```python
from build123d import *

# Parameters (mm, degrees)
SKETCH1_R           = 10
BOSS_EXTRUDE1_DEPTH = 35
SKETCH2_R           = 2.9
CUT_EXTRUDE1_DEPTH  = 12
CUT_EXTRUDE1_DRAFT  = 1
SKETCH4_R           = 2.38125
CUT_EXTRUDE2_DEPTH  = 35
SKETCH5_R           = 2.8
CUT_EXTRUDE3_DEPTH  = 38.749172176


with BuildPart() as part:
    # Sketch1 → Boss-Extrude1 (new body)
    with BuildSketch(Plane.XY):
        Circle(SKETCH1_R)
    extrude(amount=BOSS_EXTRUDE1_DEPTH)


with BuildPart() as cut_extrude1_tool:
    # Sketch2 → Cut-Extrude1 (with draft: the straight prism first)
    with BuildSketch(Plane.XY.offset(12)):
        Circle(SKETCH2_R)
    extrude(amount=-CUT_EXTRUDE1_DEPTH)
    # Cut-Extrude1: the draft: its side faces are tilted about the plane it starts from
    cut_extrude1_sides = [cut_extrude1_tool.faces().sort_by_distance(p)[0] for p in [
        (-2.9, 0, 6),
    ]]
    draft(cut_extrude1_sides, Plane.XY.offset(12), CUT_EXTRUDE1_DRAFT)


with BuildPart() as part_1:
    add(part.part)

    # Cut-Extrude1: cut by cut_extrude1_tool
    add(cut_extrude1_tool.part, mode=Mode.SUBTRACT)

    # Sketch4 → Cut-Extrude2 (cut)
    with BuildSketch(Plane.XY.offset(35)):
        Circle(SKETCH4_R)
    extrude(amount=-CUT_EXTRUDE2_DEPTH, mode=Mode.SUBTRACT)

    # Sketch5 → Cut-Extrude3 (cut, through all)
    with BuildSketch(Plane(origin=(0, 0, 0), x_dir=(1, 0, 0), z_dir=(0, 1, 0))):
        with Locations(Location((0, -7, 0), (0, 0, 90))):
            Circle(SKETCH5_R)
    extrude(amount=CUT_EXTRUDE3_DEPTH, mode=Mode.SUBTRACT)


solid = part_1.part
```
Build history of the part. All positions in model axes, mm. A direction names the side the tool comes from. Give positions to 0.01 mm unless a question says otherwise; leave off trailing zeros. Loops run counter-clockwise (first coordinate to the right, second up) from the corner with the lowest first, then second, coordinate; pieces in that order, holes last. Notation, with made-up numbers: (-37.5, 9) -> (0.5, 9) arc R6 cw to (0.5, 16) -> close; hole circle Ø4 at (17.5, 85.25). An arc over 180 degrees is marked (long way). One line per question, with ' | ' between items. Start each with the question number.
1) Pin check, flat tip, straight feed: pin 1 (3 mm diameter, centred on x = 3, z = 12.5, fed in from +Y). Stop position of the tip, or through.
2) Cut at A-A (z = 29). Give the cut face in (x, y).
3) Two-plate mould, pull along Y, no slides. Class faces 3 (the flat face through (-2.4, 2.4, 0)), 4 (the cylindrical face through (-2.17, -9.76, 17.26)), 5 (the conical face through (-0.651, -2.932, 6.084)): released by +Y, released by -Y, zero draft, split by the parting line, or undercut.
4) Cut at D-D (y = -4.5). Give the cut face in (x, z), plus the area to 3 significant figures.
5) Cut at C-C (x = 0). Count the separate pieces of the cut face and the enclosed holes in it, plus the area to 3 significant figures.
6) 3-axis set-ups, long thin cutter, end or side, ignore diameter. For faces 1 (the cylindrical face through (-0.1, 6.5, 9.8)), 2 (the flat face through (2, -2, 35)): which of +Z, -Z, +X, -X, +Y, -Y reach the whole face in a straight line?
7) Cut at B-B (y = 3.5). Give the cut face in (x, z), plus the area to 3 significant figures.
8) Probe L1, parallel to Y at x = 1.5, z = 33.5; L2, parallel to X at y = 8, z = 7; L3, parallel to X at y = 5.5, z = 7. List the from-to ranges inside material, lowest first.
Return value:
1) pin 1: y = 9.89
2) outline: circle Ø20 at (0, 0); hole circle Ø4.76 at (0, 0)
3) face 3: zero draft | face 4: split by the parting line | face 5: undercut
4) outline: (-8.93, 0) -> (8.93, 0) -> (8.93, 35) -> (-8.93, 35) -> close | area: 625 mm^2
5) separate pieces: 3 | enclosed holes: 0 | area: 479 mm^2
6) face 1: +Y | face 2: +Z, +X, -X, +Y, -Y
7) outline: (-9.37, 0) -> (9.37, 0) -> (9.37, 35) -> (-9.37, 35) -> close; hole circle Ø5.6 at (0, 7) | area: 631 mm^2
8) L1: -9.89 to -1.85, 1.85 to 9.89 | L2: -6 to -2.8, 2.8 to 6 | L3: -8.35 to -2.8, 2.8 to 8.35
